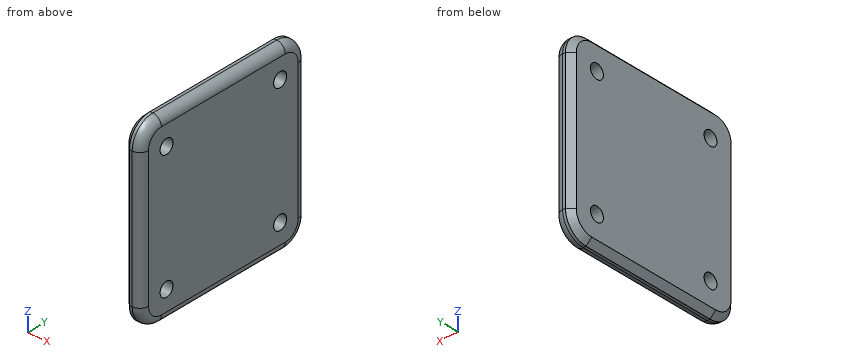
```python
from build123d import *

# Parameters (mm, degrees)
BASE_EXTRUDE_DEPTH = 9.525
CHAMFER1_SIZE      = 3.175
FILLET1_R          = 4.7752
SKETCH2_R          = 3.96875
CUT_EXTRUDE1_DEPTH = 25.4


with BuildPart() as part:
    # Sketch1 → Base-Extrude (new body)
    with BuildSketch(Plane(origin=(0, 0, 0), x_dir=(0, 0, -1), z_dir=(1, 0, 0))):
        with BuildLine():
            Line((-127, 139.7), (-50.8, 139.7))
            ThreePointArc((-50.8, 139.7), (-41.819743879, 135.980256121), (-38.1, 127))
            Line((-38.1, 127), (-38.1, 50.8))
            ThreePointArc((-38.1, 50.8), (-41.819743879, 41.819743879), (-50.8, 38.1))
            Line((-50.8, 38.1), (-127, 38.1))
            ThreePointArc((-127, 38.1), (-135.980256121, 41.819743879), (-139.7, 50.8))
            Line((-139.7, 50.8), (-139.7, 127))
            ThreePointArc((-139.7, 127), (-135.980256121, 135.980256121), (-127, 139.7))
        make_face()
    extrude(amount=BASE_EXTRUDE_DEPTH)

    # Chamfer1
    chamfer1_edges = [part.edges().sort_by_distance(p)[0] for p in [
        (0, 38.1, 88.9),
        (0, 41.819743879, 135.980256121),
        (0, 88.9, 139.7),
        (0, 135.980256121, 135.980256121),
        (0, 139.7, 88.9),
        (0, 135.980256121, 41.819743879),
        (0, 88.9, 38.1),
        (0, 41.819743879, 41.819743879),
    ]]
    chamfer(chamfer1_edges, length=CHAMFER1_SIZE)

    # Fillet1
    fillet1_edges = [part.edges().sort_by_distance(p)[0] for p in [
        (9.525, 135.980256121, 41.819743879),
        (9.525, 139.7, 88.9),
        (9.525, 135.980256121, 135.980256121),
        (9.525, 88.9, 139.7),
        (9.525, 41.819743879, 135.980256121),
        (9.525, 38.1, 88.9),
        (9.525, 41.819743879, 41.819743879),
        (9.525, 88.9, 38.1),
    ]]
    fillet(fillet1_edges, radius=FILLET1_R)

    # Sketch2 → Cut-Extrude1 (cut)
    with BuildSketch(Plane(origin=(9.525, 0, 0), x_dir=(0, 0, -1), z_dir=(1, 0, 0))):
        with Locations((-53.975, 53.975)):
            Circle(SKETCH2_R)
        with Locations((-53.975, 123.825)):
            Circle(SKETCH2_R)
        with Locations((-123.825, 123.825)):
            Circle(SKETCH2_R)
        with Locations((-123.825, 53.975)):
            Circle(SKETCH2_R)
    extrude(amount=-CUT_EXTRUDE1_DEPTH, mode=Mode.SUBTRACT)


solid = part.part
```
The listing builds one solid part. Answer for the finished solid, in the listing's coordinates (mm). Coordinates: 2 decimals unless noted, no trailing zeros. Write each loop counter-clockwise with the first axis right and the second up, starting at its lowest first coordinate (ties: lowest second). Pieces come first, ordered by that corner, then holes. Notation, with made-up numbers: M -34,52.25 L -7,52.25 A21 ccw -7,56.25 Z; hole C 59.25,86 d8. An arc over 180 degrees is marked long. Use a Markdown table: item, result. Add a question column.
1. Section A-A (y = 108) is taken. Give the vertices of the cut face in (x, z) (3 decimals).
2. Straight lines are drawn through the part: line 1 along Y through (x, z) = (6.5, 53.5); line 2 along Y through (x, z) = (2.25, 124) (3 decimals); line 3 along Z through (x, y) = (5.25, 104.5). For each, find the intervals that lie inside material, in ascending order. Write a range as [from, to].
3. Section D-D (x = 1.5) is taken. Count the separate pieces of the cut face and the enclosed holes in it, plus the area to 3 significant figures.
4. Section B-B (x = 6.75) is taken. Give the vertices of the cut face in (y, z) (1 decimal).
Data:
| question | item | result |
|---|---|---|
| 1 | outline | M 0,41.275 L 3.175,38.1 L 4.75,38.1 A4.775 ccw 9.525,42.875 L 9.525,134.925 A4.775 ccw 4.75,139.7 L 3.175,139.7 L 0,136.525 Z |
| 2 | line 1 | y = [38.43, 50.03], [57.92, 119.88], [127.77, 139.37] |
| 2 | line 2 | y = [39.025, 50.01], [57.94, 119.86], [127.79, 138.775] |
| 2 | line 3 | z = [38.13, 139.67] |
| 3 | separate pieces | 1 |
| 3 | enclosed holes | 4 |
| 3 | area | 9,350 mm2 |
| 4 | outline | M 38.5,50.8 A12.3 ccw 50.8,38.5 L 127,38.5 A12.3 ccw 139.3,50.8 L 139.3,127 A12.3 ccw 127,139.3 L 50.8,139.3 A12.3 ccw 38.5,127 Z; hole C 54,54 d7.9; hole C 54,123.8 d7.9; hole C 123.8,54 d7.9; hole C 123.8,123.8 d7.9 |
